```python
from build123d import *

# Parameters (mm, degrees)
SKETCH1_W                  = 12.7
SKETCH1_H                  = 12.7
BOSS_EXTRUDE1_DEPTH        = 25.4
SKETCH2_W                  = 6.35
SKETCH2_H                  = 6.35
BOSS_EXTRUDE2_DEPTH        = 6.35
F_10_32_TAPPED_HOLE2_D     = 4.0386
F_10_32_TAPPED_HOLE2_DEPTH = 12.7
F_10_32_TAPPED_HOLE2_TIP   = 1.213317848
F_10_32_TAPPED_HOLE3_D     = 4.0386
F_10_32_TAPPED_HOLE3_DEPTH = 12.7
F_10_32_TAPPED_HOLE3_TIP   = 1.213317848


with BuildPart() as part:
    # Sketch1 → Boss-Extrude1 (new body)
    with BuildSketch(Plane(origin=(0, 0, 0), x_dir=(1, 0, 0), z_dir=(0, 1, 0))):
        Rectangle(SKETCH1_W, SKETCH1_H)
    extrude(amount=BOSS_EXTRUDE1_DEPTH)

    # Sketch2 → Boss-Extrude2 (add)
    with BuildSketch(Plane.XZ):
        Rectangle(SKETCH2_W, SKETCH2_H)
    extrude(amount=BOSS_EXTRUDE2_DEPTH)

    # #10-32 Tapped Hole2
    with Locations(Plane(origin=(0, -6.35, 0), x_dir=(-1, 0, 0), z_dir=(0, -1, 0))):
        with Locations((0, 0)):
            Hole(F_10_32_TAPPED_HOLE2_D / 2, depth=F_10_32_TAPPED_HOLE2_DEPTH)
            with Locations((0, 0, -(F_10_32_TAPPED_HOLE2_DEPTH + F_10_32_TAPPED_HOLE2_TIP / 2))):  # 118° drill point
                Cone(0, F_10_32_TAPPED_HOLE2_D / 2, F_10_32_TAPPED_HOLE2_TIP, mode=Mode.SUBTRACT)

    # #10-32 Tapped Hole3
    with Locations(Plane(origin=(0, 25.4, 0), x_dir=(1, 0, 0), z_dir=(0, 1, 0))):
        with Locations((0, 0)):
            Hole(F_10_32_TAPPED_HOLE3_D / 2, depth=F_10_32_TAPPED_HOLE3_DEPTH)
            with Locations((0, 0, -(F_10_32_TAPPED_HOLE3_DEPTH + F_10_32_TAPPED_HOLE3_TIP / 2))):  # 118° drill point
                Cone(0, F_10_32_TAPPED_HOLE3_D / 2, F_10_32_TAPPED_HOLE3_TIP, mode=Mode.SUBTRACT)


solid = part.part
```
Source: CAD feature listing. Evaluate the final solid. Frame: model axes, mm. A direction names the side the tool comes from. Coordinates: 2 decimals unless noted, no trailing zeros. Loops run counter-clockwise (first coordinate to the right, second up) from the corner with the lowest first, then second, coordinate; pieces in that order, holes last. Notation, with made-up numbers: M 58,-8 L 106,-8 A27 cw 106,20 Z; hole C 33,86.5 d4. An arc over 180 degrees is marked long. Put each result on its own line as item: value. Start each with the question number.
1) Cut plane D-D on y = -3.5. Return the cut outline in (x, z) (3 decimals), then the cut area to 3 significant figures.
2) Ray query, L1, parallel to Z at x = 0, y = 18; L2, parallel to Z at x = 0, y = -1 (3 decimals); L3, parallel to Y at x = 4.75, z = 2. Return the intervals inside material, ascending. Write a range as from..to.
3) Contact query for flat-ended pins moving along their axis: pin 1 Ø3 at (x, y) = (0, -2) entering from -Z (3 decimals); pin 2 Ø3 at (y, z) = (-2, -1.5) entering from +X (3 decimals); pin 3 Ø3 at (x, z) = (0, 0) entering from -Y. Output: stop coordinate, or through.
4) Cut plane C-C on z = 2.75. Return the cut outline in (x, y) (3 decimals), then the cut area to 3 significant figures.
5) Cut plane B-B on y = 3. Return the cut outline in (x, z).
6) Pull-direction query (Z, two-part tool) for faces 1 (the face through (0.076, 7.353, 0.342)), 2 (the face through (0, -3, 3.175)), 3 (the face through (0, -6.35, 2.2)), 4 (the face through (0, 13, -6.35)); classes: pulls with the +Z half, pulls with the -Z half, needs draft (parallel to the pull), parting line crosses it, or undercut.
7) Reachability of faces 5 (the face through (0, -3, -3.175)), 6 (the face through (-3.175, -3, 0)), 7 (the face through (3.175, -3, 0)), 8 (the face through (1.926, 0.089, -0.607)), 9 (the face through (-1.926, 18.961, -0.607)) from +Z, -Z, +X, -X, +Y, -Y: full face, straight path, thin tool, end or side. Return the list, or none.
8) Cut plane A-A on x = 2.5. Return the cut outline in (y, z) (3 decimals), then the cut area to 3 significant figures.
The answers:
1. outline: M -3.175,-3.175 L 3.175,-3.175 L 3.175,3.175 L -3.175,3.175 Z; hole C 0,0 d4.039
1. area: 27.5 mm²
2. L1: z = -6.35..-2.02, 2.02..6.35
2. L2: z = -3.175..-2.019, 2.019..3.175
2. L3: y = 0..25.4
3. pin 1: stops at z = -3.175
3. pin 2: stops at x = 3.175
3. pin 3: stops at y = 6.66
4. outline: M -6.35,0 L -3.175,0 L -3.175,-6.35 L 3.175,-6.35 L 3.175,0 L 6.35,0 L 6.35,25.4 L -6.35,25.4 Z
4. area: 363 mm²
5. outline: M -6.35,-6.35 L 6.35,-6.35 L 6.35,6.35 L -6.35,6.35 Z; hole C 0,0 d4.04
6. face 1: undercut
6. face 2: pulls with the +Z half
6. face 3: needs draft
6. face 4: pulls with the -Z half
7. face 5: -Z, +X, -X, -Y
7. face 6: +Z, -Z, -X, -Y
7. face 7: +Z, -Z, +X, -Y
7. face 8: -Y
7. face 9: +Y
8. outline: M -6.35,-3.175 L 0,-3.175 L 0,-6.35 L 25.4,-6.35 L 25.4,6.35 L 0,6.35 L 0,3.175 L -6.35,3.175 Z
8. area: 363 mm²
